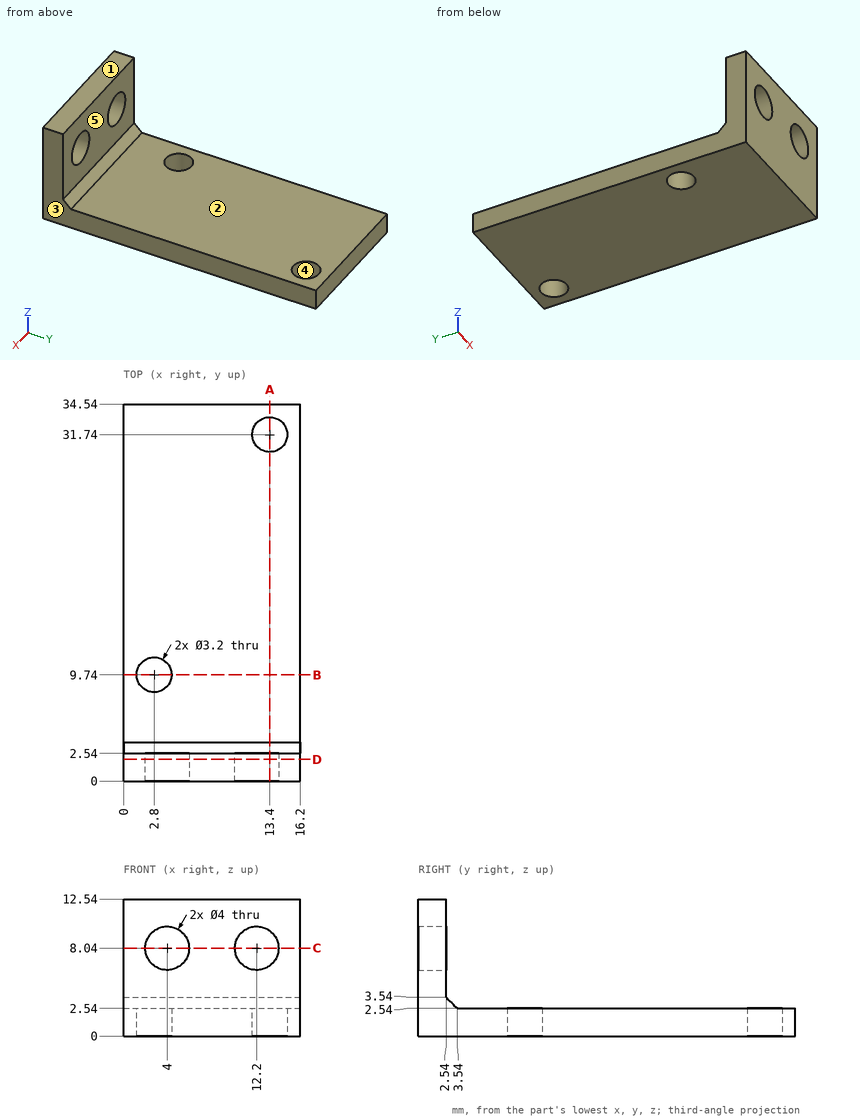
Here's the drawing with two shaded views (mm, measured from the low corner). I have some questions. A direction names the side the tool comes from. Give positions to 0.01 mm unless a question says otherwise; leave off trailing zeros. Order: outer loops, then holes, each group sorted by start corner. A loop starts at its lowest first (then second) coordinate and runs counter-clockwise, first axis right, second up. Notation, with made-up numbers: M -22,48.5 L 32,48.5 A30 ccw 32,79.5 Z; hole C 55,29 d2. An arc over 180 degrees is marked long. Answer as a JSON object with one key per item and string values. Group by question number.
1) Suppose I cut it at C-C, the plane z = 8.04. Write out the boundary of the cut face in (x, y), plus the area to 3 significant figures.
2) Suppose I cut it at D-D, the plane y = 2. Write out the boundary of the cut face in (x, z), plus the area to 3 significant figures.
3) Suppose I cut it at B-B, the plane y = 9.74. Write out the boundary of the cut face in (x, z).
4) Suppose I cut it at A-A, the plane x = 13.4. Write out the boundary of the cut face in (y, z), plus the area to 3 significant figures.
5) We'd pull the mould along Y, two halves only. Please class the marked faces 3, 4 and 5: pulls with the +Y half, pulls with the -Y half, needs draft (parallel to the pull), parting line crosses it, or undercut.
6) On a 3-axis mill with a long thin cutter (end or side, diameter ignored), from which of +Z, -Z, +X, -X, +Y, -Y can I reach the whole of each face in a straight line? I mean the marked faces 1 and 2. Say none if no direction works.
7) I'm going to push flat-ended pins straight in: pin 1 Ø2.5 at (x, z) = (11.5, 9) entering from +Y; pin 2 Ø5 at (x, y) = (8.5, 26.5) entering from +Z. Where does each tip first touch, or does it pass through?
8) Please list where these lines run through material, in increasing order: L1, parallel to X at y = 0.65, z = 8.04; L2, parallel to Z at x = 4, y = 1.35; L3, parallel to Y at x = 13.4, z = 1.25. Write a range as [from, to].
Results found:
{
 "1": {"outline": "M 0,0 L 2,0 L 2,2.54 L 0,2.54 Z; M 6,0 L 10.2,0 L 10.2,2.54 L 6,2.54 Z; M 14.2,0 L 16.2,0 L 16.2,2.54 L 14.2,2.54 Z", "area": "20.8 mm²"},
 "2": {"outline": "M 0,0 L 16.2,0 L 16.2,12.54 L 0,12.54 Z; hole C 4,8.04 d4; hole C 12.2,8.04 d4", "area": "178 mm²"},
 "3": {"outline": "M 0,0 L 1.2,0 L 1.2,2.54 L 0,2.54 Z; M 4.4,0 L 16.2,0 L 16.2,2.54 L 4.4,2.54 Z"},
 "4": {"outline": "M 0,0 L 30.14,0 L 30.14,2.54 L 3.54,2.54 L 2.54,3.54 L 2.54,6.44 L 0,6.44 Z; M 0,9.64 L 2.54,9.64 L 2.54,12.54 L 0,12.54 Z; M 33.34,0 L 34.54,0 L 34.54,2.54 L 33.34,2.54 Z", "area": "97.4 mm²"},
 "5": {"face 3": "needs draft", "face 4": "undercut", "face 5": "pulls with the +Y half"},
 "6": {"face 1": "+Z, +X, -X, +Y, -Y", "face 2": "+Z, +X, -X, +Y"},
 "7": {"pin 1": "y = 2.54", "pin 2": "z = 2.54"},
 "8": {"L1": "[0, 2], [6, 10.2], [14.2, 16.2]", "L2": "[0, 6.04], [10.04, 12.54]", "L3": "[0, 30.14], [33.34, 34.54]"}
}
